CAD build for the part. Positions are in the model's coordinates, mm. A direction names the side the tool comes from. Give positions to 0.01 mm unless a question says otherwise; leave off trailing zeros. Order: outer loops, then holes, each group sorted by start corner. A loop starts at its lowest first (then second) coordinate and runs counter-clockwise, first axis right, second up.
Item 1: Which spindle directions (+Z, -Z, +X, -X, +Y, -Y) get a long thin tool onto all of the face, cutting with end or side? Do faces 5 (the flat face through (-6, 3, 7.5)), 6 (the flat face through (4, 2, -3)), 7 (the flat face through (-4, 4, -4)), 8 (the flat face through (6.6, 2, -3)). Say none if no direction does.
Item 2: Two-plate mould, pull along Z, no slides. Class faces 1 (the flat face through (-6, 3, 4.5)), 2 (the flat face through (0, 2, -7.5)), 3 (the flat face through (-6, 3, 4)), 4 (the flat face through (-5.603, 2, -4)): released by +Z, released by -Z, zero draft, split by the parting line, or undercut.
Item 3: Flat gauge pins, fed straight in: P1, Ø1.2, axis at x = 0, y = 1.5, coming from the -Z side; P2, Ø1.5, axis at x = -4.5, y = 2.5, coming from the -Z side; P3, Ø1.8, axis at x = -5, z = -4.5, coming from the +Y side. Where does each tip first touch, or does it go through?
Item 4: Band-saw the part on B-B on z = -16.5. Give the cut face in (x, y), plus the area to 3 significant figures.
Item 5: Band-saw the part on A-A on x = -0.5. Give the cut face in (y, z), plus the area to 3 significant figures.
Item 6: Wall check: L1, parallel to Z at x = -4.25, y = 1.45; L2, parallel to Y at x = -0.25, z = -9; L3, parallel to Z at x = -6, y = 0.7. Give the ranges that are in metal, low to high.
```python
from build123d import *

# Parameters (mm, degrees)
SKETCH1_W           = 16
SKETCH1_H           = 20
BOSS_EXTRUDE1_DEPTH = 1
SKETCH2_W           = 4
SKETCH2_H           = 2.5
BOSS_EXTRUDE2_DEPTH = 3.5
SKETCH3_W           = 5
SKETCH3_H           = 5
SKETCH3_W_2         = 2.6
SKETCH3_H_2         = 4
BOSS_EXTRUDE3_DEPTH = 1.5
SKETCH4_W           = 2.302574488
SKETCH4_H           = 3
BOSS_EXTRUDE4_DEPTH = 3
SKETCH5_R           = 0.2
BOSS_EXTRUDE5_DEPTH = 78


with BuildPart() as part:
    # Sketch1 → Boss-Extrude1 (new body)
    with BuildSketch(Plane(origin=(0, 0, 0), x_dir=(1, 0, 0), z_dir=(0, 1, 0))):
        Rectangle(SKETCH1_W, SKETCH1_H)
    extrude(amount=BOSS_EXTRUDE1_DEPTH)

    # Sketch2 → Boss-Extrude2 (add)
    with BuildSketch(Plane(origin=(0, 1, 0), x_dir=(1, 0, 0), z_dir=(0, 1, 0))):
        with Locations((-6, -5.75)):
            Rectangle(SKETCH2_W, SKETCH2_H)
        with Locations((-6, -8.75)):
            Rectangle(SKETCH2_W, SKETCH2_H)
        with Locations((-6, -2.75)):
            Rectangle(SKETCH2_W, SKETCH2_H)
        with Locations((6, -5.75)):
            Rectangle(SKETCH2_W, SKETCH2_H)
    extrude(amount=BOSS_EXTRUDE2_DEPTH)

    # Sketch3 → Boss-Extrude3 (add)
    with BuildSketch(Plane(origin=(0, 1, 0), x_dir=(1, 0, 0), z_dir=(0, 1, 0))):
        with Locations((0, 5)):
            Rectangle(SKETCH3_W, SKETCH3_H)
        with Locations((5.3, 3.5)):
            Rectangle(SKETCH3_W_2, SKETCH3_H_2)
    extrude(amount=BOSS_EXTRUDE3_DEPTH)

    # Sketch4 → Boss-Extrude4 (add)
    with BuildSketch(Plane(origin=(0, 1, 0), x_dir=(1, 0, 0), z_dir=(0, 1, 0))):
        with Locations((-4.451287244, 4)):
            Rectangle(SKETCH4_W, SKETCH4_H)
    extrude(amount=BOSS_EXTRUDE4_DEPTH)

    # Sketch5 → Boss-Extrude5 (add)
    with BuildSketch(Plane(origin=(0, 0, -10), x_dir=(-1, 0, 0), z_dir=(0, 0, -1))):
        with Locations(Location((7.4, 0.5, 0), (0, 0, 180))):
            Circle(SKETCH5_R)
        with Locations(Location((-7.4, 0.5, 0), (0, 0, 180))):
            Circle(SKETCH5_R)
    extrude(amount=BOSS_EXTRUDE5_DEPTH)


solid = part.part
```
The answers:
1. face 5: +X, -X, +Y
1. face 6: +Z, -Z, +Y
1. face 7: -Z, +X, -X, +Y
1. face 8: -Z, +X, +Y
2. face 1: undercut
2. face 2: released by -Z
2. face 3: undercut
2. face 4: zero draft
3. P1: stops at z = -10
3. P2: stops at z = -5.5
3. P3: stops at y = 4
4. outline: circle Ø0.4 at (-7.4, 0.5); circle Ø0.4 at (7.4, 0.5)
4. area: 0.251 mm2
5. outline: (0, -10) - (1, -10) - (1, -7.5) - (2.5, -7.5) - (2.5, -2.5) - (1, -2.5) - (1, 10) - (0, 10) - close
5. area: 27.5 mm2
6. L1: z = -5.5 to -2.5, 1.5 to 4, 4.5 to 7, 7.5 to 10
6. L2: y = 0 to 1
6. L3: z = -10 to 10
